Check sheet for the modelled part. Datum: model origin and axes. Units: mm. A direction names the side the tool comes from. Round coordinates to 2 decimals unless told otherwise and drop trailing zeros. Write each loop counter-clockwise with the first axis right and the second up, starting at its lowest first coordinate (ties: lowest second). Pieces come first, ordered by that corner, then holes. Notation, with made-up numbers: M 10.5,7 L 21.5,7 A17 ccw 21.5,35 Z; hole C 58,84 d11. An arc over 180 degrees is marked long. Answer in a Markdown table with one row per item.
```python
from build123d import *

# Parameters (mm, degrees)
BOSS_EXTRUDE1_DEPTH                            = 8
BOSS_EXTRUDE2_DEPTH                            = 40
SKETCH1_4_W                                    = 8
SKETCH1_4_H                                    = 20
BOSS_EXTRUDE3_DEPTH                            = 2
RIB3_REACH                                     = 72.887
SKETCH3_WALL_W                                 = 167.227880054
SKETCH3_WALL_H                                 = 2
FILLET2_R                                      = 3
BOSS_EXTRUDE4_DEPTH                            = 64
SKETCH5_W                                      = 86
SKETCH5_H                                      = 78
BOSS_EXTRUDE5_DEPTH                            = 6.5
FILLET3_R                                      = 10
CSK_FOR_8_FLAT_HEAD_MACHINE_SCREW1_D           = 4.4958
CSK_FOR_8_FLAT_HEAD_MACHINE_SCREW1_CSINK_D     = 8.4328
CSK_FOR_8_FLAT_HEAD_MACHINE_SCREW1_CSINK_ANGLE = 82
FILLET4_R                                      = 2
RIB4_REACH                                     = 102.29
SKETCH7_WALL_W                                 = 223.792364866
SKETCH7_WALL_H                                 = 2
LPATTERN1_COUNT                                = 3
LPATTERN1_PITCH                                = 10
LPATTERN1_COL_COUNT                            = 3
LPATTERN1_COL_PITCH                            = 10
MIRROR3_COPY_1_REACH                           = 102.29
MIRROR3_COPY_1_SKETCH_W                        = 223.792364866
MIRROR3_COPY_1_SKETCH_H                        = 2
MIRROR3_COPY_2_REACH                           = 102.29
MIRROR3_COPY_2_SKETCH_W                        = 223.792364866
MIRROR3_COPY_2_SKETCH_H                        = 2
MIRROR3_COPY_3_REACH                           = 102.29
MIRROR3_COPY_3_SKETCH_W                        = 223.792364866
MIRROR3_COPY_3_SKETCH_H                        = 2
MIRROR3_COPY_4_REACH                           = 102.29
MIRROR3_COPY_4_SKETCH_W                        = 223.792364866
MIRROR3_COPY_4_SKETCH_H                        = 2
RIB5_REACH                                     = 105.315
SKETCH8_WALL_W                                 = 229.843307728
SKETCH8_WALL_H                                 = 2
LPATTERN2_COUNT                                = 3
LPATTERN2_PITCH                                = 8
LPATTERN2_COL_COUNT                            = 3
LPATTERN2_COL_PITCH                            = 8
MIRROR4_COPY_1_REACH                           = 105.315
MIRROR4_COPY_1_SKETCH_W                        = 229.843307728
MIRROR4_COPY_1_SKETCH_H                        = 2
MIRROR4_COPY_2_REACH                           = 105.315
MIRROR4_COPY_2_SKETCH_W                        = 229.843307728
MIRROR4_COPY_2_SKETCH_H                        = 2
MIRROR4_COPY_3_REACH                           = 105.315
MIRROR4_COPY_3_SKETCH_W                        = 229.843307728
MIRROR4_COPY_3_SKETCH_H                        = 2
MIRROR4_COPY_4_REACH                           = 105.315
MIRROR4_COPY_4_SKETCH_W                        = 229.843307728
MIRROR4_COPY_4_SKETCH_H                        = 2


with BuildPart() as part:
    # Sketch1 → Boss-Extrude1 (new body)
    with BuildSketch(Plane.XY):
        Polygon((40, 0), (0, 0), (-8, 0), (-8, -8), (48, -8), (48, 0), align=None)
    extrude(amount=BOSS_EXTRUDE1_DEPTH)

    # Sketch1<3> → Boss-Extrude2 (add)
    with BuildSketch(Plane.XY):
        Polygon((40, 0), (0, 0), (-8, 0), (-8, -8), (48, -8), (48, 0), align=None)
    extrude(amount=-BOSS_EXTRUDE2_DEPTH)

    # Sketch1<4> → Boss-Extrude3 (add)
    with BuildSketch(Plane.XY):
        with Locations((-4, 10)):
            Rectangle(SKETCH1_4_W, SKETCH1_4_H)
        with Locations((44, 10)):
            Rectangle(SKETCH1_4_W, SKETCH1_4_H)
    extrude(amount=-BOSS_EXTRUDE3_DEPTH)

    # Sketch3 wall → Rib3 (add, up to next)
    with BuildSketch(Plane(origin=(-7, 10, -8.125), x_dir=(0, -0.852754414843, -0.522312079092), z_dir=(0, -0.522312079092, 0.852754414843)), mode=Mode.PRIVATE) as rib3_sk1:
        with Locations((0, 1)):
            Rectangle(SKETCH3_WALL_W, SKETCH3_WALL_H)
    rib3_tool1 = extrude(rib3_sk1.sketch, amount=RIB3_REACH, mode=Mode.PRIVATE) - part.part
    rib3 = rib3_tool1.solids().sort_by_distance((-7, 10, -8.125))[0]
    add(rib3)

    # Mirror2: Rib3 across plane
    add(rib3.mirror(Plane.ZY.offset(-20)))

    # Fillet2
    fillet2_edges = [part.edges().sort_by_distance(p)[0] for p in [
        (-8, -4, 8),
        (-8, -4, -40),
        (48, -4, -40),
        (48, -4, 8),
    ]]
    fillet(fillet2_edges, radius=FILLET2_R)

    # Sketch4 → Boss-Extrude4 (add)
    with BuildSketch(Plane.XZ.offset(8)):
        with BuildLine():
            Line((-5, -40), (45, -40))
            ThreePointArc((45, -40), (47.121320344, -39.121320344), (48, -37))
            Line((48, -37), (48, 5))
            ThreePointArc((48, 5), (47.121320344, 7.121320344), (45, 8))
            Line((45, 8), (-5, 8))
            ThreePointArc((-5, 8), (-7.121320344, 7.121320344), (-8, 5))
            Line((-8, 5), (-8, -37))
            ThreePointArc((-8, -37), (-7.121320344, -39.121320344), (-5, -40))
        make_face()
    extrude(amount=BOSS_EXTRUDE4_DEPTH)

    # Sketch5 → Boss-Extrude5 (add)
    with BuildSketch(Plane.XZ.offset(72)):
        with Locations((20, -16)):
            Rectangle(SKETCH5_W, SKETCH5_H)
    extrude(amount=-BOSS_EXTRUDE5_DEPTH)

    # Fillet3
    fillet3_edges = [part.edges().sort_by_distance(p)[0] for p in [
        (-23, -68.75, -55),
        (-23, -68.75, 23),
        (63, -68.75, 23),
        (63, -68.75, -55),
    ]]
    fillet(fillet3_edges, radius=FILLET3_R)

    # CSK for #8 Flat Head Machine Screw1 (through all)
    with Locations(Plane(origin=(-13, -65.5, 13), x_dir=(1, 0, 0), z_dir=(0, 1, 0))):
        with Locations((0, 0), (0, 58), (66, 0), (66, 58)):
            CounterSinkHole(CSK_FOR_8_FLAT_HEAD_MACHINE_SCREW1_D / 2, CSK_FOR_8_FLAT_HEAD_MACHINE_SCREW1_CSINK_D / 2, counter_sink_angle=CSK_FOR_8_FLAT_HEAD_MACHINE_SCREW1_CSINK_ANGLE)

    # Fillet4
    fillet4_edges = [part.edges().sort_by_distance(p)[0] for p in [
        (-7.121320344, -65.5, -39.121320344),
        (20, -65.5, -40),
        (-8, -65.5, -16),
        (48, -65.5, -16),
        (47.121320344, -65.5, 7.121320344),
        (20, -65.5, 8),
        (-7.121320344, -65.5, 7.121320344),
        (47.121320344, -65.5, -39.121320344),
    ]]
    fillet(fillet4_edges, radius=FILLET4_R)

    # Sketch7 wall → Rib4 (add, up to next)
    with BuildSketch(Plane(origin=(20, -58, -47.5), x_dir=(0, 0.707106781187, 0.707106781187), z_dir=(0, 0.707106781187, -0.707106781187)), mode=Mode.PRIVATE) as rib4_sk1:
        Rectangle(SKETCH7_WALL_W, SKETCH7_WALL_H)
    rib4_tool1 = extrude(rib4_sk1.sketch, amount=-RIB4_REACH, mode=Mode.PRIVATE) - part.part
    rib4 = rib4_tool1.solids().sort_by_distance((20, -58, -47.5))[0]
    add(rib4)

    # LPattern1: Rib4 ×3
    with Locations(*[(-i * LPATTERN1_PITCH, 0, 0) for i in range(1, LPATTERN1_COUNT)]):
        add(rib4)

    # LPattern1 col: Rib4 ×3
    with Locations(*[(i * LPATTERN1_COL_PITCH, 0, 0) for i in range(1, LPATTERN1_COL_COUNT)]):
        add(rib4)

    # Mirror3: Rib4 across plane
    add(rib4.mirror(Plane(origin=(0, 0, -16), x_dir=(1, 0, 0), z_dir=(0, 0, -1))))

    # Mirror3 copy 1 sketch → Mirror3 copy 1 (add, up to next)
    with BuildSketch(Plane(origin=(10, -58, 15.5), x_dir=(0, 0.707106781187, -0.707106781187), z_dir=(0, 0.707106781187, 0.707106781187)), mode=Mode.PRIVATE) as mirror3_copy_1_sk1:
        Rectangle(MIRROR3_COPY_1_SKETCH_W, MIRROR3_COPY_1_SKETCH_H)
    mirror3_copy_1_tool1 = extrude(mirror3_copy_1_sk1.sketch, amount=-MIRROR3_COPY_1_REACH, mode=Mode.PRIVATE) - part.part
    add(mirror3_copy_1_tool1.solids().sort_by_distance((10, -58, 15.5))[0])

    # Mirror3 copy 2 sketch → Mirror3 copy 2 (add, up to next)
    with BuildSketch(Plane(origin=(0, -58, 15.5), x_dir=(0, 0.707106781187, -0.707106781187), z_dir=(0, 0.707106781187, 0.707106781187)), mode=Mode.PRIVATE) as mirror3_copy_2_sk1:
        Rectangle(MIRROR3_COPY_2_SKETCH_W, MIRROR3_COPY_2_SKETCH_H)
    mirror3_copy_2_tool1 = extrude(mirror3_copy_2_sk1.sketch, amount=-MIRROR3_COPY_2_REACH, mode=Mode.PRIVATE) - part.part
    add(mirror3_copy_2_tool1.solids().sort_by_distance((0, -58, 15.5))[0])

    # Mirror3 copy 3 sketch → Mirror3 copy 3 (add, up to next)
    with BuildSketch(Plane(origin=(30, -58, 15.5), x_dir=(0, 0.707106781187, -0.707106781187), z_dir=(0, 0.707106781187, 0.707106781187)), mode=Mode.PRIVATE) as mirror3_copy_3_sk1:
        Rectangle(MIRROR3_COPY_3_SKETCH_W, MIRROR3_COPY_3_SKETCH_H)
    mirror3_copy_3_tool1 = extrude(mirror3_copy_3_sk1.sketch, amount=-MIRROR3_COPY_3_REACH, mode=Mode.PRIVATE) - part.part
    add(mirror3_copy_3_tool1.solids().sort_by_distance((30, -58, 15.5))[0])

    # Mirror3 copy 4 sketch → Mirror3 copy 4 (add, up to next)
    with BuildSketch(Plane(origin=(40, -58, 15.5), x_dir=(0, 0.707106781187, -0.707106781187), z_dir=(0, 0.707106781187, 0.707106781187)), mode=Mode.PRIVATE) as mirror3_copy_4_sk1:
        Rectangle(MIRROR3_COPY_4_SKETCH_W, MIRROR3_COPY_4_SKETCH_H)
    mirror3_copy_4_tool1 = extrude(mirror3_copy_4_sk1.sketch, amount=-MIRROR3_COPY_4_REACH, mode=Mode.PRIVATE) - part.part
    add(mirror3_copy_4_tool1.solids().sort_by_distance((40, -58, 15.5))[0])

    # Sketch8 wall → Rib5 (add, up to next)
    with BuildSketch(Plane(origin=(-15.5, -58, -16), x_dir=(-0.707106781187, -0.707106781187, 0), z_dir=(-0.707106781187, 0.707106781187, 0)), mode=Mode.PRIVATE) as rib5_sk1:
        Rectangle(SKETCH8_WALL_W, SKETCH8_WALL_H)
    rib5_tool1 = extrude(rib5_sk1.sketch, amount=-RIB5_REACH, mode=Mode.PRIVATE) - part.part
    rib5 = rib5_tool1.solids().sort_by_distance((-15.5, -58, -16))[0]
    add(rib5)

    # LPattern2: Rib5 ×3
    with Locations(*[(0, 0, -i * LPATTERN2_PITCH) for i in range(1, LPATTERN2_COUNT)]):
        add(rib5)

    # LPattern2 col: Rib5 ×3
    with Locations(*[(0, 0, i * LPATTERN2_COL_PITCH) for i in range(1, LPATTERN2_COL_COUNT)]):
        add(rib5)

    # Mirror4: Rib5 across plane
    add(rib5.mirror(Plane.ZY.offset(-20)))

    # Mirror4 copy 1 sketch → Mirror4 copy 1 (add, up to next)
    with BuildSketch(Plane(origin=(55.5, -58, -24), x_dir=(0.707106781187, -0.707106781187, 0), z_dir=(0.707106781187, 0.707106781187, 0)), mode=Mode.PRIVATE) as mirror4_copy_1_sk1:
        Rectangle(MIRROR4_COPY_1_SKETCH_W, MIRROR4_COPY_1_SKETCH_H)
    mirror4_copy_1_tool1 = extrude(mirror4_copy_1_sk1.sketch, amount=-MIRROR4_COPY_1_REACH, mode=Mode.PRIVATE) - part.part
    add(mirror4_copy_1_tool1.solids().sort_by_distance((55.5, -58, -24))[0])

    # Mirror4 copy 2 sketch → Mirror4 copy 2 (add, up to next)
    with BuildSketch(Plane(origin=(55.5, -58, -32), x_dir=(0.707106781187, -0.707106781187, 0), z_dir=(0.707106781187, 0.707106781187, 0)), mode=Mode.PRIVATE) as mirror4_copy_2_sk1:
        Rectangle(MIRROR4_COPY_2_SKETCH_W, MIRROR4_COPY_2_SKETCH_H)
    mirror4_copy_2_tool1 = extrude(mirror4_copy_2_sk1.sketch, amount=-MIRROR4_COPY_2_REACH, mode=Mode.PRIVATE) - part.part
    add(mirror4_copy_2_tool1.solids().sort_by_distance((55.5, -58, -32))[0])

    # Mirror4 copy 3 sketch → Mirror4 copy 3 (add, up to next)
    with BuildSketch(Plane(origin=(55.5, -58, -8), x_dir=(0.707106781187, -0.707106781187, 0), z_dir=(0.707106781187, 0.707106781187, 0)), mode=Mode.PRIVATE) as mirror4_copy_3_sk1:
        Rectangle(MIRROR4_COPY_3_SKETCH_W, MIRROR4_COPY_3_SKETCH_H)
    mirror4_copy_3_tool1 = extrude(mirror4_copy_3_sk1.sketch, amount=-MIRROR4_COPY_3_REACH, mode=Mode.PRIVATE) - part.part
    add(mirror4_copy_3_tool1.solids().sort_by_distance((55.5, -58, -8))[0])

    # Mirror4 copy 4 sketch → Mirror4 copy 4 (add, up to next)
    with BuildSketch(Plane(origin=(55.5, -58, 0), x_dir=(0.707106781187, -0.707106781187, 0), z_dir=(0.707106781187, 0.707106781187, 0)), mode=Mode.PRIVATE) as mirror4_copy_4_sk1:
        Rectangle(MIRROR4_COPY_4_SKETCH_W, MIRROR4_COPY_4_SKETCH_H)
    mirror4_copy_4_tool1 = extrude(mirror4_copy_4_sk1.sketch, amount=-MIRROR4_COPY_4_REACH, mode=Mode.PRIVATE) - part.part
    add(mirror4_copy_4_tool1.solids().sort_by_distance((55.5, -58, 0))[0])


solid = part.part
```
1. Section check A-A, the plane y = -4. Record the cut outline in (x, z).
Found:
| item | result |
|---|---|
| outline | M -8,-37 A3 ccw -5,-40 L 45,-40 A3 ccw 48,-37 L 48,5 A3 ccw 45,8 L -5,8 A3 ccw -8,5 Z |
2. Access from +Z, -Z, +X, -X, +Y, -Y to the whole of each face (thin tool, end or side, straight path). Record for faces 4 (the face through (21, -61, 13)), 5 (the face through (25, -65.5, -48)), 6 (the face through (-10, -65.5, -41)), 7 (the face through (47.1, -31.31, -39.14)), 8 (the face through (-13, -61, -15)).
Found:
| item | result |
|---|---|
| face 4 | +Z, +Y |
| face 5 | -Z, +Y |
| face 6 | -Z, -X, +Y |
| face 7 | -Z, +X, +Y |
| face 8 | -X, +Y |
3. Draft check along X on faces 1 (the face through (56, -65.5, -12)), 2 (the face through (55.4, -57.9, 0)), 3 (the face through (39, -61, 13)). Enter one of: +X half, -X half, draft (parallel to the pull), parting line (faces both ways), or undercut.
Found:
| item | result |
|---|---|
| face 1 | draft |
| face 2 | +X half |
| face 3 | undercut |
4. Go/stop test with flat-tipped pins: pin 1 (5 mm diameter, centred on x = 2.5, y = -19.5, fed in from +Z); pin 2 (7.5 mm diameter, centred on x = -14, y = -61, fed in from +Z); pin 3 (3 mm diameter, centred on x = 0.5, z = -1, fed in from +Y); pin 4 (12 mm diameter, centred on y = -54.5, z = 15.5, fed in from +X). Record where each tip stops, or that it passes through.
Found:
| item | result |
|---|---|
| pin 1 | stops at z = 8 |
| pin 2 | stops at z = 1 |
| pin 3 | stops at y = 20 |
| pin 4 | stops at x = 41 |
5. Section check B-B, the plane x = 4.5. Record the cut outline in (y, z), and give its area (3 significant figures).
Found:
| item | result |
|---|---|
| outline | M -72,-55 L -65.5,-55 L -65.5,-42 A2 cw -63.5,-40 L 0,-40 L 0,8 L -63.5,8 A2 cw -65.5,10 L -65.5,23 L -72,23 Z |
| area | 3,650 mm2 |
6. Scan lines: L1, parallel to X at y = -68, z = -45; L2, parallel to Z at x = -13, y = -70.9; L3, parallel to Y at x = 23, z = 18.5. Record each from-to range of solid material in increasing order.
Found:
| item | result |
|---|---|
| L1 | x = -23 to -15.25, -10.75 to 50.75, 55.25 to 63 |
| L2 | z = -55 to -47.25, -42.75 to 10.75, 15.25 to 23 |
| L3 | y = -72 to -65.5 |
